Drawing for the job (mm, zero at the part's lowest x, y, z). A direction names the side the tool comes from. Round coordinates to 2 decimals unless told otherwise and drop trailing zeros. Write each loop counter-clockwise with the first axis right and the second up, starting at its lowest first coordinate (ties: lowest second). Pieces come first, ordered by that corner, then holes.
Item 1: Band-saw the part on B-B, the plane x = 66. Write the cut outline in (y, z).
Item 2: 3-axis set-ups, long thin cutter, end or side, ignore diameter. For the marked faces 1 and 2: which of +Z, -Z, +X, -X, +Y, -Y reach the whole face in a straight line?
Item 3: Drop flat-ended pins along their axis: pin 1 Ø8.5 at (x, y) = (82, 5.5) entering from +Z; pin 2 Ø12 at (x, z) = (125, 190.5) entering from -Y. Give the stop position or say it passes through.
Item 4: Wall check: probe 1 along X at (y, z) = (4, 76.5); probe 2 along Y at (x, z) = (37, 135); probe 3 along Z at (x, y) = (123, 10.5). Give the ranges that are in metal, low to high.
Item 5: Band-saw the part on C-C, the plane z = 26. Write the cut outline in (x, y).
Item 6: Band-saw the part on A-A, the plane y = 11. Write the cut outline in (x, z) (1 decimal), then the cut area to 3 significant figures.
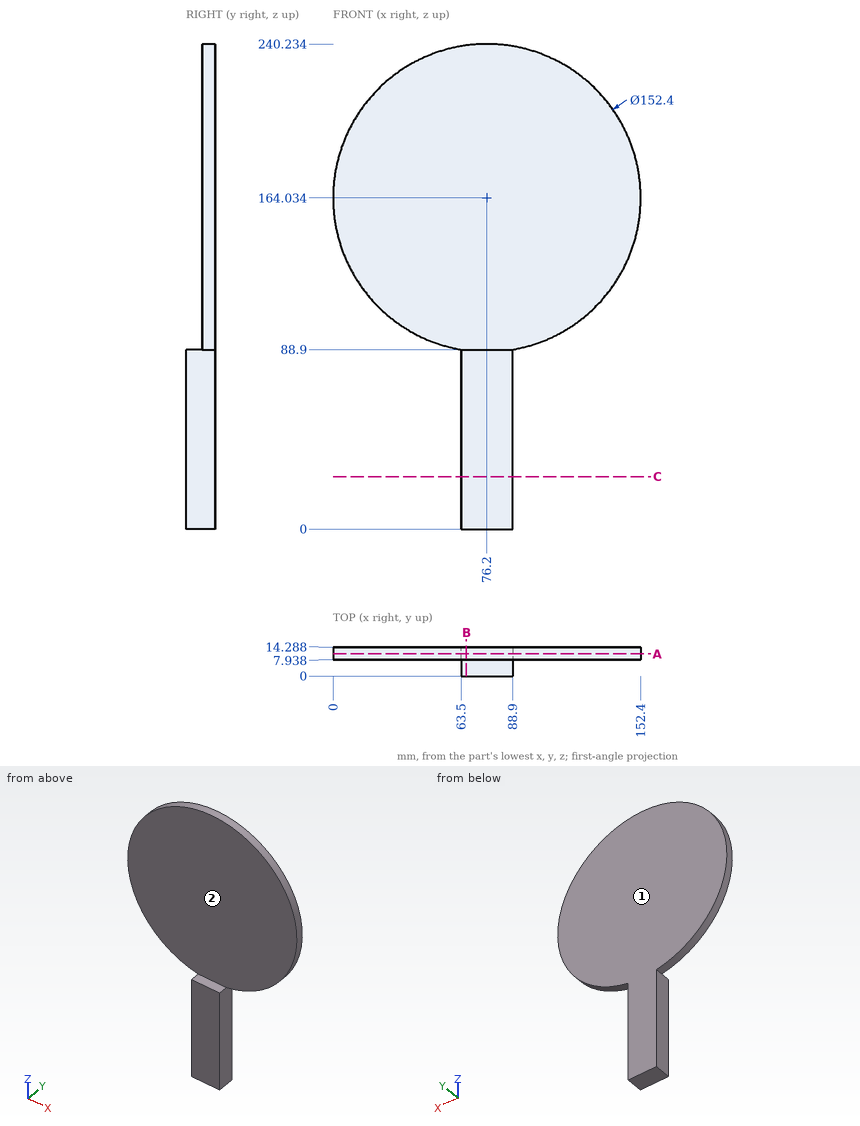
Results:
1. outline: (0, 0) - (14.29, 0) - (14.29, 239.55) - (7.94, 239.55) - (7.94, 88.9) - (0, 88.9) - close
2. face 1: +Z, -Z, +X, -X, +Y
2. face 2: +Z, +X, -X, -Y
3. pin 1: stops at z = 240.2
3. pin 2: stops at y = 7.94
4. probe 1: x = 63.5 to 88.9
4. probe 2: y = 7.94 to 14.29
4. probe 3: z = 103.9 to 224.17
5. outline: (63.5, 0) - (88.9, 0) - (88.9, 14.29) - (63.5, 14.29) - close
6. outline: (63.5, 0) - (88.9, 0) - (88.9, 88.9) arc R76.2 ccw (long way) to (63.5, 88.9) - close
6. area: 20,500 mm2
